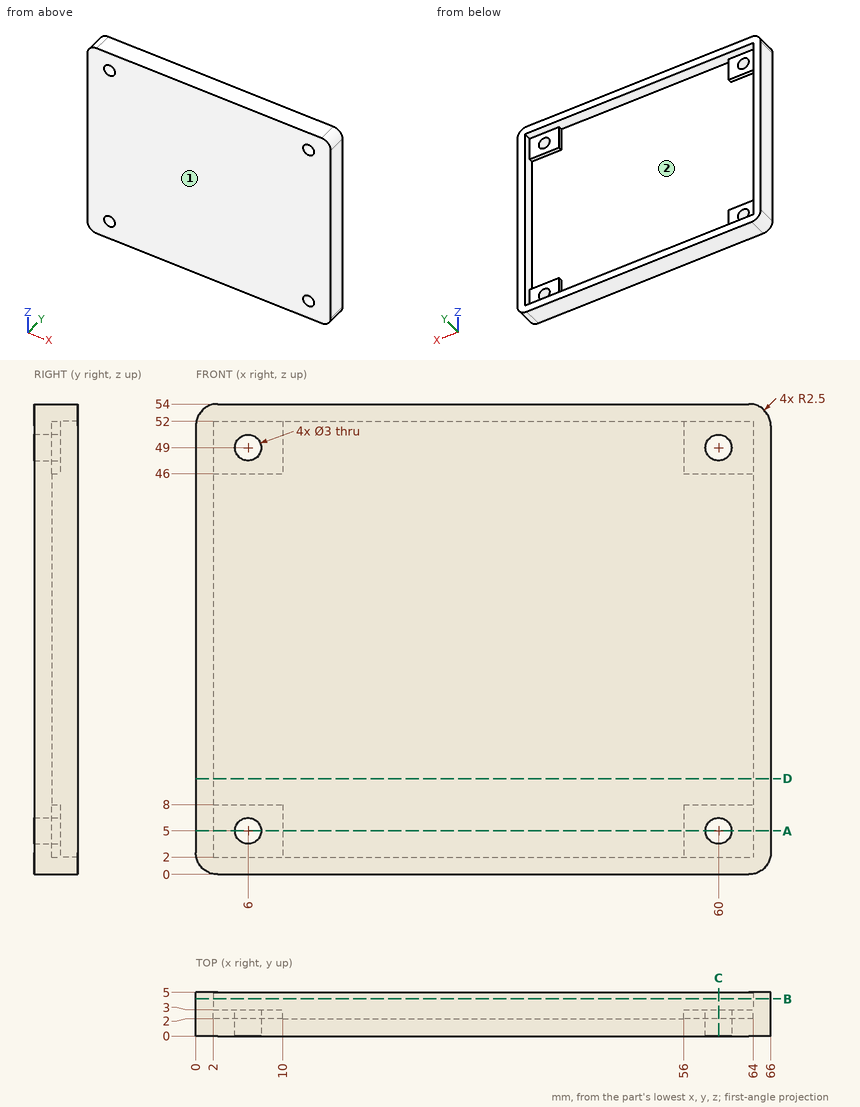
Study the drawing (mm; zero at the part's minimum x, y, z) and answer. Round coordinates to 2 decimals unless told otherwise and drop trailing zeros. Write each loop counter-clockwise with the first axis right and the second up, starting at its lowest first coordinate (ties: lowest second). Pieces come first, ordered by that corner, then holes. Notation, with made-up numbers: (-34.5, 54) -> (-11.5, 54) arc R24 ccw to (-11.5, 78) -> close; hole circle Ø5 at (37, -7). An arc over 180 degrees is marked (long way). Write each question's results on one line, items separated by ' | '.
Item 1: A cutting plane is placed at D-D, the plane z = 11. Determine the outline of the cut face in (x, y), plus the area to 3 significant figures.
Result set:
outline: (0, 0) -> (66, 0) -> (66, 5) -> (64, 5) -> (64, 2) -> (2, 2) -> (2, 5) -> (0, 5) -> close | area: 144 mm^2
Item 2: The mould has two halves that part along X. Classify the marked faces 1 and 2: +X half, -X half, draft (parallel to the pull), parting line (faces both ways), or undercut.
Result set:
face 1: draft | face 2: undercut
Item 3: A cutting plane is placed at C-C, the plane x = 60. Determine the outline of the cut face in (y, z), plus the area to 3 significant figures.
Result set:
outline: (0, 0) -> (5, 0) -> (5, 2) -> (3, 2) -> (3, 3.5) -> (0, 3.5) -> close; (0, 6.5) -> (3, 6.5) -> (3, 8) -> (2, 8) -> (2, 46) -> (3, 46) -> (3, 47.5) -> (0, 47.5) -> close; (0, 50.5) -> (3, 50.5) -> (3, 52) -> (5, 52) -> (5, 54) -> (0, 54) -> close | area: 114 mm^2
Item 4: A cutting plane is placed at B-B, the plane y = 4.25. Determine the outline of the cut face in (x, z), plus the area to 3 significant figures.
Result set:
outline: (0, 2.5) arc R2.5 ccw to (2.5, 0) -> (63.5, 0) arc R2.5 ccw to (66, 2.5) -> (66, 51.5) arc R2.5 ccw to (63.5, 54) -> (2.5, 54) arc R2.5 ccw to (0, 51.5) -> close; hole (2, 2) -> (64, 2) -> (64, 52) -> (2, 52) -> close | area: 459 mm^2
Item 5: A cutting plane is placed at A-A, the plane z = 5. Determine the outline of the cut face in (x, y), plus the area to 3 significant figures.
Result set:
outline: (0, 0) -> (4.5, 0) -> (4.5, 3) -> (2, 3) -> (2, 5) -> (0, 5) -> close; (7.5, 0) -> (58.5, 0) -> (58.5, 3) -> (56, 3) -> (56, 2) -> (10, 2) -> (10, 3) -> (7.5, 3) -> close; (61.5, 0) -> (66, 0) -> (66, 5) -> (64, 5) -> (64, 3) -> (61.5, 3) -> close | area: 142 mm^2
Item 6: Find the intervals of material crossed by line 1 along X through (y, z) = (1.05, 5); line 2 along Z through (x, y) = (60, 1.2); line 3 along Z through (x, y) = (6, 2.2), in increasing order. Write a range as [from, to].
Result set:
line 1: [0, 4.5], [7.5, 58.5], [61.5, 66] | line 2: [0, 3.5], [6.5, 47.5], [50.5, 54] | line 3: [0, 3.5], [6.5, 8], [46, 47.5], [50.5, 54]
Item 7: Flat-ended cylindrical pins translate along their axes: P1, Ø0.5, axis at y = 2.5, z = 4, coming from the -X side; P2, Ø5, axis at x = 60, z = 5, coming from the +Y side; P3, Ø1, axis at x = 35, z = 10.5, coming from the +Y side. Find the tip coordinate at first contact, or state that the pin passes through.
Result set:
P1: x = 0 | P2: y = 3 | P3: y = 2
